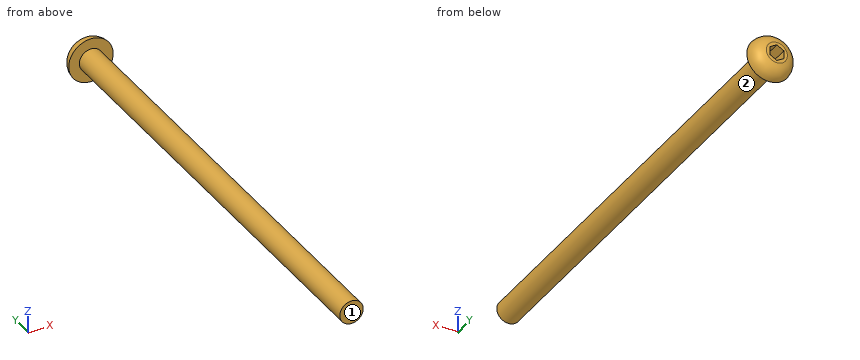
```python
from build123d import *

# Parameters (mm, degrees)
F0_R     = 2.5
F1_DEPTH = 100
F5_DEPTH = 4


with BuildPart() as f1:
    # F0 (on Front) → F1 (new body)
    with BuildSketch(Plane.XZ):
        Circle(F0_R)
    extrude(amount=F1_DEPTH)

    # F2 (on Right) → F3 (revolve)
    with BuildSketch(Plane.YZ):
        with BuildLine():
            Line((0, 4.75), (0, 0))
            Line((0, 0), (3, 0))
            Line((3, 0), (3, 1.5))
            Line((3, 1.5), (3, 2.25))
            ThreePointArc((3, 2.25), (1.952562, 4.043075), (0, 4.75))
        make_face()
    revolve(axis=Axis((0, 0, 0), (0, -1, 0)))

    # F4 (on face) → F5 (cut)
    with BuildSketch(Plane(origin=(0, 3, 0), x_dir=(-1, 0, 0), z_dir=(0, 1, 0))):
        Polygon((-1.5, 0.866025), (-1.5, -0.866025), (0, -1.732051), (1.5, -0.866025), (1.5, 0.866025), (0, 1.732051), align=None)
    extrude(amount=-F5_DEPTH, mode=Mode.SUBTRACT)


solid = f1.part
```
Model file for the job. Use its own axes, mm. Face numbers are marked on the shaded views. A direction names the side the tool comes from. Coordinates: 2 decimals unless noted, no trailing zeros. Write each loop counter-clockwise with the first axis right and the second up, starting at its lowest first coordinate (ties: lowest second). Pieces come first, ordered by that corner, then holes. Notation, with made-up numbers: (-27.5, 51) - (-0.5, 51) arc R25 ccw to (-0.5, 79) - close; hole circle Ø4 at (0, -34.5). An arc over 180 degrees is marked (long way). One line per question, with ' | ' between items. Start each with the question number.
Q1. 3-axis set-ups, long thin cutter, end or side, ignore diameter. For the marked faces 1 and 2: which of +Z, -Z, +X, -X, +Y, -Y reach the whole face in a straight line?
Q2. Cut at A-A, the plane y = -62. List the corners of the cut face in (x, z), then the cut area to 3 significant figures.
Q3. Drill centre lines: line 1 (Y direction, x = 0.5, z = -0.5); line 2 (X direction, y = -38, z = -2); line 3 (Y direction, x = -1.5, z = -1.75). Where is each one in solid material? Low to high. Write a range as [from, to].
Q4. Pin check, flat tips, straight feed: pin 1 (3 mm diameter, centred on y = -22.5, z = 2.5, fed in from +X); pin 2 (5 mm diameter, centred on x = 1.5, y = -68.5, fed in from -Z). Stop position of each tip, or through.
Answer below:
1) face 1: +Z, -Z, +X, -X, -Y | face 2: -Y
2) outline: circle Ø5 at (0, 0) | area: 19.6 mm^2
3) line 1: [-100, -1] | line 2: [-1.5, 1.5] | line 3: [-100, 2.99]
4) pin 1: x = 2.29 | pin 2: z = -2.5
